Geometry: see drawing. Coordinates: mm, zero at the bounding-box minimum. A direction names the side the tool comes from. Round coordinates to 2 decimals unless told otherwise and drop trailing zeros. Loops run counter-clockwise (first coordinate to the right, second up) from the corner with the lowest first, then second, coordinate; pieces in that order, holes last. Notation, with made-up numbers: (6.25, -30.75) -> (47.25, -30.75) arc R25 cw to (47.25, 8.25) -> close; hole circle Ø11 at (49.25, 40). An arc over 180 degrees is marked (long way). Write item = value, one per line.
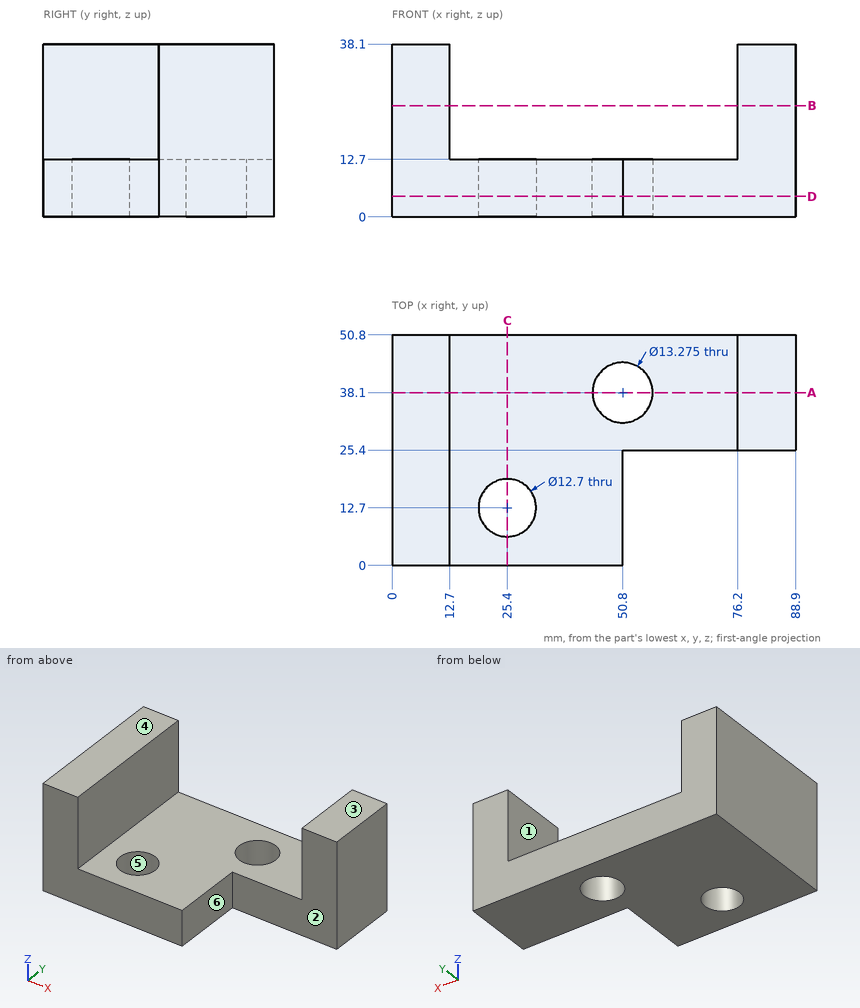
1. Section query A-A (y = 38.1). Return the cut outline in (x, z).
Evaluation:
outline = (0, 0) -> (44.16, 0) -> (44.16, 12.7) -> (12.7, 12.7) -> (12.7, 38.1) -> (0, 38.1) -> close; (57.44, 0) -> (88.9, 0) -> (88.9, 38.1) -> (76.2, 38.1) -> (76.2, 12.7) -> (57.44, 12.7) -> close
2. Section query B-B (z = 24.5). Return the cut outline in (x, y).
Evaluation:
outline = (0, 0) -> (12.7, 0) -> (12.7, 50.8) -> (0, 50.8) -> close; (76.2, 25.4) -> (88.9, 25.4) -> (88.9, 50.8) -> (76.2, 50.8) -> close
3. Section query C-C (x = 25.4). Return the cut outline in (y, z), then the cut area to 3 significant figures.
Evaluation:
outline = (0, 0) -> (6.35, 0) -> (6.35, 12.7) -> (0, 12.7) -> close; (19.05, 0) -> (50.8, 0) -> (50.8, 12.7) -> (19.05, 12.7) -> close
area = 484 mm²
4. Set-up query: the marked faces 1, 2 and 3. Return all of +Z, -Z, +X, -X, +Y, -Y with unobstructed straight access to the full face (end or side cutting, diameter ignored); none if empty.
Evaluation:
face_1 = +Z, +Y, -Y
face_2 = +Z, -Z, +X, -Y
face_3 = +Z, +X, -X, +Y, -Y
5. Mould query, pull axis X, two halves, no side actions, for the marked faces 4, 5 and 6. Classes: released by +X, released by -X, zero draft, split by the parting line, or undercut.
Evaluation:
face_4 = zero draft
face_5 = undercut
face_6 = released by +X
6. Line query: probe 1 along Y at (x, z) = (25, 10); probe 2 along X at (y, z) = (32, 33.5); probe 3 along Y at (x, z) = (60.5, 8). Output: solid intervals per line, ascending. Write a range as from..to.
Evaluation:
probe_1 = 0..6.36, 19.04..50.8
probe_2 = 0..12.7, 76.2..88.9
probe_3 = 25.4..50.8
7. Section query D-D (z = 4.5). Give the number of separate pieces and of enclosed holes in the cut face, then the cut area to 3 significant figures.
Evaluation:
separate_pieces = 1
enclosed_holes = 2
area = 3,280 mm²
8. Contact query for flat-ended pins moving along their axis: pin 1 Ø11.5 at (x, y) = (25.4, 12.7) entering from +Z; pin 2 Ø10 at (y, z) = (11, 9) entering from +X; pin 3 Ø6 at (y, z) = (21.5, 19) entering from +X. Output: stop coordinate, or through.
Evaluation:
pin_1 = through
pin_2 = 50.8
pin_3 = 12.7
